```python
from build123d import *

# Parameters (mm, degrees)
F0_R            = 1.75
F1_DEPTH        = 12
F3_DEPTH        = 2
F4_W            = 50
F4_H            = 12.016664
F5_DEPTH        = 2
F6_R            = 1.1
F7_DEPTH        = 60
F9_DEPTH        = 11
F11_DEPTH       = 11
F13_D           = 2.2
F13_DEPTH       = 3
F13_CSINK_D     = 4
F13_CSINK_ANGLE = 90
F15_D           = 2.2
F15_DEPTH       = 3
F15_CSINK_D     = 4
F15_CSINK_ANGLE = 90
F17_DEPTH       = 25


with BuildPart() as f1:
    # F0 (on Front) → F1 (new body)
    with BuildSketch(Plane.XZ):
        with BuildLine():
            Line((0, 45), (0, 0))
            Line((0, 0), (50, 0))
            Line((50, 0), (50, 15.500001))
            Line((50, 15.500001), (45, 20.500001))
            Line((45, 20.500001), (38.5, 20.500001))
            Line((38.5, 20.500001), (34.995267, 24.004733))
            Line((34.995267, 24.004733), (25.995267, 24.004733))
            ThreePointArc((25.995267, 24.004733), (17.995267, 32.004733), (25.995267, 40.004733))
            Line((25.995267, 40.004733), (33.097442, 40.004733))
            Line((33.097442, 40.004733), (36, 43))
            Line((36, 43), (36, 48))
            Line((36, 48), (37.5, 50.5))
            Line((37.5, 50.5), (37.5, 55))
            Line((37.5, 55), (10, 55))
            ThreePointArc((10, 55), (2.928932, 52.071068), (0, 45))
        make_face()
        with Locations((10, 5)):
            Circle(F0_R, mode=Mode.SUBTRACT)
        with BuildLine():
            ThreePointArc((12, 17.546566), (13.5, 16.046566), (12, 14.546566))
            Line((12, 14.546566), (8, 14.546566))
            ThreePointArc((8, 14.546566), (6.5, 16.046566), (8, 17.546566))
            Line((8, 17.546566), (12, 17.546566))
        make_face(mode=Mode.SUBTRACT)
        with Locations((40, 5)):
            Circle(F0_R, mode=Mode.SUBTRACT)
        with BuildLine():
            ThreePointArc((43.990533, 17.500001), (45.490533, 16.000001), (43.990533, 14.500001))
            Line((43.990533, 14.500001), (39.990533, 14.500001))
            ThreePointArc((39.990533, 14.500001), (38.490533, 16.000001), (39.990533, 17.500001))
            Line((39.990533, 17.500001), (43.990533, 17.500001))
        make_face(mode=Mode.SUBTRACT)
        with BuildLine():
            ThreePointArc((12, 49.5), (13.5, 48), (12, 46.5))
            Line((12, 46.5), (8, 46.5))
            ThreePointArc((8, 46.5), (6.5, 48), (8, 49.5))
            Line((8, 49.5), (12, 49.5))
        make_face(mode=Mode.SUBTRACT)
    extrude(amount=F1_DEPTH)

    # F2 (on face) → F3 (cut)
    with BuildSketch(Plane(origin=(0, 0, 0), x_dir=(-1, 0, 0), z_dir=(0, 1, 0))):
        with BuildLine():
            Line((-38.5, 20.005015), (-26.077409, 20.005015))
            ThreePointArc((-26.077409, 20.005015), (-13.995267, 32.0056), (-26.079143, 44.00444))
            Line((-26.079143, 44.00444), (-36, 44.00444))
            Line((-36, 44.00444), (-38.5, 44.00444))
            Line((-38.5, 44.00444), (-38.5, 20.500001))
            Line((-38.5, 20.500001), (-38.5, 20.005015))
        make_face()
    extrude(amount=-F3_DEPTH, mode=Mode.SUBTRACT)

    # F4 (on face) → F5 (cut)
    with BuildSketch(Plane(origin=(0, 0, 0), x_dir=(-1, 0, 0), z_dir=(0, 1, 0))):
        with Locations((-25, 6.008332)):
            Rectangle(F4_W, F4_H)
    extrude(amount=-F5_DEPTH, mode=Mode.SUBTRACT)

    # F6 (on face) → F7 (cut)
    with BuildSketch(Plane.XY.offset(55)):
        with Locations((32.499979, -7)):
            Circle(F6_R)
    extrude(amount=-F7_DEPTH, mode=Mode.SUBTRACT)

    # F8 (on face) → F9 (cut)
    with BuildSketch(Plane.YZ.offset(50)):
        with BuildLine():
            ThreePointArc((-7, 9.25), (-5.762563, 9.762563), (-5.25, 11))
            ThreePointArc((-5.25, 11), (-8.237437, 12.237437), (-7, 9.25))
        make_face()
    extrude(amount=-F9_DEPTH, mode=Mode.SUBTRACT)

    # F10 (on face) → F11 (cut)
    with BuildSketch(Plane(origin=(0, 0, 0), x_dir=(-1, 0, 0), z_dir=(0, 1, 0))):
        Polygon((-44, 14), (-44, 11), (-43.990533, 8), (-41, 8), (-41, 14), align=None)
    extrude(amount=-F11_DEPTH, mode=Mode.SUBTRACT)

    # F13
    with Locations(Plane.XY.offset(24.004733)):
        with Locations((32.499979, -7)):
            CounterSinkHole(F13_D / 2, F13_CSINK_D / 2, depth=F13_DEPTH, counter_sink_angle=F13_CSINK_ANGLE)

    # F15
    with Locations(Plane.XY.offset(55)):
        with Locations((32.499979, -7)):
            CounterSinkHole(F15_D / 2, F15_CSINK_D / 2, depth=F15_DEPTH, counter_sink_angle=F15_CSINK_ANGLE)

    # F16 (on face) → F17 (cut)
    with BuildSketch(Plane.XZ.offset(12)):
        with BuildLine():
            Line((45.717547, 19.782453), (45.717547, 20.859413))
            ThreePointArc((45.717547, 20.859413), (39.79599, 35.138554), (41.570501, 19.782453))
            Line((41.570501, 19.782453), (41.944866, 19.782453))
            Line((41.944866, 19.782453), (45.717547, 19.782453))
        make_face()
        with BuildLine():
            Line((41.944866, 19.782453), (41.570501, 19.782453))
            ThreePointArc((41.570501, 19.782453), (41.757683, 19.780208), (41.944866, 19.782453))
        make_face()
    extrude(amount=-F17_DEPTH, mode=Mode.SUBTRACT)


solid = f1.part
```
Geometry: final body of the model. Coordinates: model frame, mm. A direction names the side the tool comes from. Coordinates: 2 decimals unless noted, no trailing zeros. Order: outer loops, then holes, each group sorted by start corner. A loop starts at its lowest first (then second) coordinate and runs counter-clockwise, first axis right, second up.
Item 1: Section query A-A (z = 5). Output: boundary loops of the cut face in (x, y).
Answer:
outline: (0, -12) - (8.25, -12) - (8.25, -2) - (0, -2) - close; (11.75, -12) - (38.25, -12) - (38.25, -2) - (11.75, -2) - close; (41.75, -12) - (50, -12) - (50, -2) - (41.75, -2) - close; hole circle Ø2.2 at (32.5, -7)
Item 2: Access query for faces 1 (the face through (31, -1, 44.004)), 2 (the face through (6.5, -5.9, 48)), 3 (the face through (21, -1, 12.017)), 4 (the face through (36, -6, 45)). Directions: +Z, -Z, +X, -X, +Y, -Y. A direction counts if a zero-diameter tool reaches every point of the face in a straight line with its end or side. Return the directions, or none.
Answer:
face 1: +X, +Y
face 2: +Y, -Y
face 3: -Z, +X, -X, +Y
face 4: +X, +Y, -Y
Item 3: Contact query for flat-ended pins moving along their axis: P1, Ø12, axis at x = 24, z = 31, coming from the +Y side; P2, Ø7, axis at x = 31.5, z = 29.5, coming from the +Y side; P3, Ø3, axis at x = 44.5, y = -4.5, coming from the +Z side; P4, Ø1.5, axis at x = 39.5, y = -2, coming from the +Z side. Output: stop coordinate, or through.
Answer:
P1: stops at y = -2
P2: passes through
P3: stops at z = 19.78
P4: stops at z = 20.38
Item 4: Draft query along X for faces 5 (the face through (3.01, -5.92, 52.15)), 6 (the face through (47, -1, 12.017)), 7 (the face through (44, -5, 13)). Return one class per face: released by +X, released by -X, zero draft, split by the parting line, or undercut.
Answer:
face 5: released by -X
face 6: zero draft
face 7: undercut
Item 5: Section query C-C (z = 51.5). Output: boundary loops of the cut face in (x, y), then the cut area to 3 significant figures.
Answer:
outline: (2.4, -12) - (37.5, -12) - (37.5, 0) - (2.4, 0) - close; hole circle Ø2.2 at (32.5, -7)
area: 417 mm2
Item 6: Section query B-B (x = 22.5). Output: boundary loops of the cut face in (y, z), then the cut area to 3 significant figures.
Answer:
outline: (-12, 0) - (-2, 0) - (-2, 12.02) - (0, 12.02) - (0, 20.53) - (-2, 20.53) - (-2, 24.81) - (-12, 24.81) - close; (-12, 39.2) - (-2, 39.2) - (-2, 43.48) - (0, 43.48) - (0, 55) - (-12, 55) - close
area: 446 mm2
Item 7: Material intervals for line 1 along Z through (x, y) = (32.5, -1.5); line 2 along Z through (x, y) = (10, -4.5); line 3 along Y through (x, z) = (45, 11), sorted ascending.
Answer:
line 1: z = 12.02 to 20.01, 44 to 55
line 2: z = 0 to 3.25, 6.75 to 14.55, 17.55 to 46.5, 49.5 to 55
line 3: y = -12 to -8.75, -5.25 to -2
